```python
from build123d import *

# Parameters (mm, degrees)
SKETCH1_W           = 9.2
SKETCH1_H           = 4
BOSS_EXTRUDE1_DEPTH = 22
SHELL1_T            = -0.5
SKETCH2_2_R         = 0.75
BOSS_EXTRUDE2_DEPTH = 22


with BuildPart() as part:
    # Sketch1 → Boss-Extrude1 (new body)
    with BuildSketch(Plane(origin=(0, 0, 0), x_dir=(0, 0, -1), z_dir=(1, 0, 0))):
        Rectangle(SKETCH1_W, SKETCH1_H)
    extrude(amount=BOSS_EXTRUDE1_DEPTH)

    # Shell1
    shell1_openings = [part.faces().sort_by_distance(p)[0] for p in [
        (0, 0, 0),
    ]]
    offset(amount=SHELL1_T, openings=shell1_openings, kind=Kind.INTERSECTION)

    # Sketch2_2 → Boss-Extrude2 (add)
    with BuildSketch(Plane(origin=(22, 0, 0), x_dir=(0, 0, -1), z_dir=(1, 0, 0))):
        Circle(SKETCH2_2_R)
        with Locations(Location((-1.6, 0, 0), (0, 0, 180))):
            Circle(SKETCH2_2_R)
        with Locations(Location((1.6, 0, 0), (0, 0, 180))):
            Circle(SKETCH2_2_R)
    extrude(amount=BOSS_EXTRUDE2_DEPTH)


solid = part.part
```
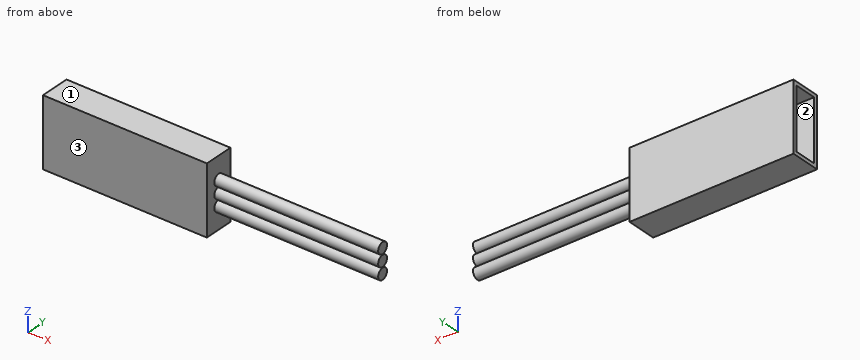
Build history of the part. All positions in model axes, mm. Face numbers are marked on the shaded views. Give positions to 0.01 mm unless a question says otherwise; leave off trailing zeros. Loops run counter-clockwise (first coordinate to the right, second up) from the corner with the lowest first, then second, coordinate; pieces in that order, holes last. Notation, with made-up numbers: (62, -39.75) -> (70, -39.75) arc R27 ccw to (70, -0.75) -> close; hole circle Ø10 at (-17.75, -35). An arc over 180 degrees is marked (long way). One line per question, with ' | ' between items. Start each with the question number.
1) Cut at A-A (z = 3.5). Give the cut face in (x, y).
2) Two-plate mould, pull along Z, no slides. Class the marked faces 1, 2 and 3: released by +Z, released by -Z, zero draft, split by the parting line, or undercut.
3) Cut at B-B (x = 10.5). Give the cut face in (y, z), plus the area to 3 significant figures.
4) Cut at D-D (z = 1.6). Give the cut face in (x, y), plus the area to 3 significant figures.
5) Cut at C-C (x = 26). Give the cut face in (y, z), plus the area to 3 significant figures.
6) Pin check, flat tips, straight feed: pin 1 (4 mm diameter, centred on x = 36, z = -2.5, fed in from -Y); pin 2 (1.5 mm diameter, centred on y = 0, z = -2, fed in from -X); pin 3 (1.5 mm diameter, centred on x = 36, z = 2.5, fed in from +Y). Stop position of each tip, or through.
7) Probe L1, parallel to Z at x = 27, y = 0.2; L2, parallel to Z at x = 2.5, y = 0.4; L3, parallel to Y at x = 6, z = -1.5. List the from-to ranges inside material, lowest first.
Return value:
1) outline: (0, -2) -> (22, -2) -> (22, 2) -> (0, 2) -> (0, 1.5) -> (21.5, 1.5) -> (21.5, -1.5) -> (0, -1.5) -> close
2) face 1: released by +Z | face 2: undercut | face 3: zero draft
3) outline: (-2, -4.6) -> (2, -4.6) -> (2, 4.6) -> (-2, 4.6) -> close; hole (-1.5, -4.1) -> (1.5, -4.1) -> (1.5, 4.1) -> (-1.5, 4.1) -> close | area: 12.2 mm^2
4) outline: (0, -2) -> (22, -2) -> (22, -0.75) -> (44, -0.75) -> (44, 0.75) -> (22, 0.75) -> (22, 2) -> (0, 2) -> (0, 1.5) -> (21.5, 1.5) -> (21.5, -1.5) -> (0, -1.5) -> close | area: 56.5 mm^2
5) outline: circle Ø1.5 at (0, -1.6); circle Ø1.5 at (0, 0); circle Ø1.5 at (0, 1.6) | area: 5.30 mm^2
6) pin 1: y = -0.75 | pin 2: x = 21.5 | pin 3: y = 0.73
7) L1: -2.32 to -0.88, -0.72 to 0.72, 0.88 to 2.32 | L2: -4.6 to -4.1, 4.1 to 4.6 | L3: -2 to -1.5, 1.5 to 2
